Verification items for the finished model (mm, model axes). Face numbers are marked on the shaded views. A direction names the side the tool comes from. Coordinates: 2 decimals unless noted, no trailing zeros. Write each loop counter-clockwise with the first axis right and the second up, starting at its lowest first coordinate (ties: lowest second). Pieces come first, ordered by that corner, then holes. Notation, with made-up numbers: (-11, -8) -> (36, -8) arc R33 cw to (36, 21) -> close; hole circle Ø8 at (31.5, 7.25). An arc over 180 degrees is marked (long way). Use CSV: the item, a comma, the result in double quotes.
```python
from build123d import *

# Parameters (mm, degrees)
TABAN_FLAN_1_DEPTH    = 535
KES_EKSTR_ZYON1_DEPTH = 10
M5_DI_LI_DELIK1_D     = 4.2
M5_DI_LI_DELIK2_D     = 4.2
M5_DI_LI_DELIK3_D     = 4.2
IZIM13_R              = 10
IZIM13_R_2            = 5
KES_EKSTR_ZYON2_DEPTH = 10


# Sheet-metal steps are written as plain solids
with BuildPart() as part:
    # Çizim1 → Taban-Flanş1 (new, symmetric)
    with BuildSketch(Plane(origin=(0, 0, 0), x_dir=(0, 0, -1), z_dir=(1, 0, 0))):
        with BuildLine():
            Line((-15, -32.5), (-3.7366, -32.5))
            ThreePointArc((-3.7366, -32.5), (-1.094424801, -31.405575199), (0, -28.7634))
            Line((0, -28.7634), (0, 28.7634))
            ThreePointArc((0, 28.7634), (-1.094424801, 31.405575199), (-3.7366, 32.5))
            Line((-3.7366, 32.5), (-15, 32.5))
            Line((-15, 32.5), (-15, 29.5))
            Line((-15, 29.5), (-3.7366, 29.5))
            ThreePointArc((-3.7366, 29.5), (-3.215745145, 29.284254855), (-3, 28.7634))
            Line((-3, 28.7634), (-3, -28.7634))
            ThreePointArc((-3, -28.7634), (-3.215745145, -29.284254855), (-3.7366, -29.5))
            Line((-3.7366, -29.5), (-15, -29.5))
            Line((-15, -29.5), (-15, -32.5))
        make_face()
    extrude(amount=TABAN_FLAN_1_DEPTH, both=True)

    # Çizim6 → Kes-Ekstrüzyon1 (cut)
    with BuildSketch(Plane(origin=(0, 0, 0), x_dir=(-1, 0, 0), z_dir=(0, 0, -1))):
        with BuildLine():
            Line((-500, 7), (-475, 7))
            ThreePointArc((-475, 7), (-468, 0), (-475, -7))
            Line((-475, -7), (-500, -7))
            ThreePointArc((-500, -7), (-507, 0), (-500, 7))
        make_face()
    extrude(amount=-KES_EKSTR_ZYON1_DEPTH, mode=Mode.SUBTRACT)

    # M5 Dişli Delik1 (through all)
    with Locations(Plane(origin=(440, 12.5, 0), x_dir=(-1, 0, 0), z_dir=(0, 0, -1))):
        with Locations((0, 0), (0, -25)):
            Hole(M5_DI_LI_DELIK1_D / 2)

    # M5 Dişli Delik2 (through all)
    with Locations(Plane(origin=(385, 10, 0), x_dir=(-1, 0, 0), z_dir=(0, 0, -1))):
        with Locations((0, 0), (0, -20)):
            m5_di_li_delik2 = Hole(M5_DI_LI_DELIK2_D / 2)

    # M5 Dişli Delik3 (through all)
    with Locations(Plane(origin=(335, 12.5, 0), x_dir=(-1, 0, 0), z_dir=(0, 0, -1))):
        with Locations((0, 0), (0, -25)):
            m5_di_li_delik3 = Hole(M5_DI_LI_DELIK3_D / 2)

    # Aynalama1: M5 Dişli Delik2, M5 Dişli Delik3 across plane
    add(m5_di_li_delik2.mirror(Plane(origin=(0, 0, 0), x_dir=(0, 0, 1), z_dir=(1, 0, 0))), mode=Mode.SUBTRACT)
    add(m5_di_li_delik3.mirror(Plane(origin=(0, 0, 0), x_dir=(0, 0, 1), z_dir=(1, 0, 0))), mode=Mode.SUBTRACT)

    # Çizim13 → Kes-Ekstrüzyon2 (cut)
    with BuildSketch(Plane(origin=(0, 0, 0), x_dir=(-1, 0, 0), z_dir=(0, 0, -1))):
        with Locations((470, 0)):
            Circle(IZIM13_R)
        with Locations((515, 20.289920322)):
            Circle(IZIM13_R_2)
        with Locations((425, -20.289920322)):
            Circle(IZIM13_R_2)
    extrude(amount=-KES_EKSTR_ZYON2_DEPTH, mode=Mode.SUBTRACT)


solid = part.part
```
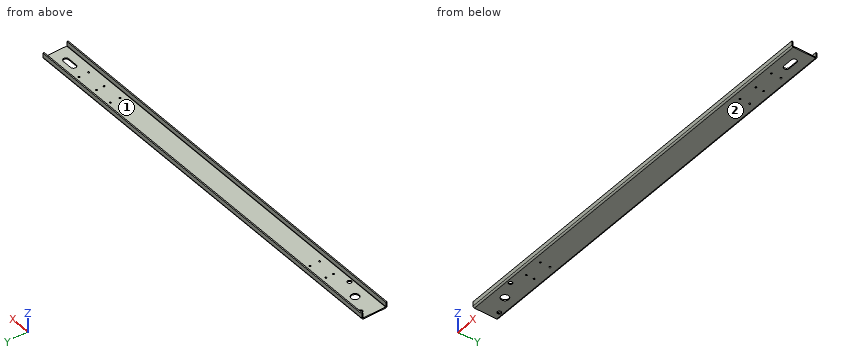
1) Cross-section at C-C (x = -7). Record the boundary of the cut face in (y, z).
Return value:
outline,"(-32.5, 3.74) arc R3.74 ccw to (-28.76, 0) -> (28.76, 0) arc R3.74 ccw to (32.5, 3.74) -> (32.5, 15) -> (29.5, 15) -> (29.5, 3.74) arc R0.74 cw to (28.76, 3) -> (-28.76, 3) arc R0.74 cw to (-29.5, 3.74) -> (-29.5, 15) -> (-32.5, 15) -> close"
2) Cross-section at B-B (z = 9). Record the boundary of the cut face in (x, y).
Return value:
outline,"(-535, -32.5) -> (535, -32.5) -> (535, -29.5) -> (-535, -29.5) -> close; (-535, 29.5) -> (535, 29.5) -> (535, 32.5) -> (-535, 32.5) -> close"
3) Cross-section at A-A (x = -470). Record the boundary of the cut face in (y, z).
Return value:
outline,"(-32.5, 3.74) arc R3.74 ccw to (-28.76, 0) -> (-10, 0) -> (-10, 3) -> (-28.76, 3) arc R0.74 cw to (-29.5, 3.74) -> (-29.5, 15) -> (-32.5, 15) -> close; (10, 0) -> (28.76, 0) arc R3.74 ccw to (32.5, 3.74) -> (32.5, 15) -> (29.5, 15) -> (29.5, 3.74) arc R0.74 cw to (28.76, 3) -> (10, 3) -> close"
4) Scan lines: L1, parallel to Y at x = -386.5, z = 2.5; L2, parallel to Y at x = -356.5, z = 5.75; L3, parallel to Y at x = -335, z = 1. Record each from-to range of solid material in increasing order.
Return value:
L1,"-32.29 to -11.47, -8.53 to 8.53, 11.47 to 32.29"
L2,"-32.5 to -29.5, 29.5 to 32.5"
L3,"-31.31 to -14.6, -10.4 to 10.4, 14.6 to 31.31"
5) Gauge pin test, flat ends, axial feed: pin 1 (12 mm diameter, centred on x = 302, y = -6.5, fed in from +Z); pin 2 (2.5 mm diameter, centred on x = -335, y = -12.5, fed in from +Z); pin 3 (3.5 mm diameter, centred on x = 489, z = 1.5, fed in from -Y); pin 4 (2.5 mm diameter, centred on x = 490.5, z = 2, fed in from +Y). Record the tip position at first contact, or that the pin passes through.
Return value:
pin 1,"z = 3"
pin 2,"through"
pin 3,"y = -32.47"
pin 4,"y = 32.47"
6) Set-up check for the marked faces 1 and 2: record each of +Z, -Z, +X, -X, +Y, -Y from which the full face is reachable in a straight line by a thin tool's end or side.
Return value:
face 1,"+Z, +X, -X"
face 2,"-Z, +X, -X, +Y, -Y"
